from build123d import *

# Parameters (mm, degrees)
F1_DEPTH = 6.35


with BuildPart() as f1:
    # F0 (on Front) → F1 (new body)
    with BuildSketch(Plane.XZ):
        with BuildLine():
            Line((254, 6.35), (0, 6.35))
            Line((0, 6.35), (0, 0))
            ThreePointArc((0, 0), (2.54, -2.54), (5.08, 0))
            Line((5.08, 0), (5.6896, 0))
            ThreePointArc((5.6896, 0), (8.2296, -2.54), (10.7696, 0))
            Line((10.7696, 0), (11.3792, 0))
            ThreePointArc((11.3792, 0), (13.9192, -2.54), (16.4592, 0))
            Line((16.4592, 0), (17.0688, 0))
            ThreePointArc((17.0688, 0), (19.6088, -2.54), (22.1488, 0))
            Line((22.1488, 0), (22.7584, 0))
            ThreePointArc((22.7584, 0), (25.2984, -2.54), (27.8384, 0))
            Line((27.8384, 0), (28.448, 0))
            ThreePointArc((28.448, 0), (30.988, -2.54), (33.528, 0))
            Line((33.528, 0), (34.1376, 0))
            ThreePointArc((34.1376, 0), (36.6776, -2.54), (39.2176, 0))
            Line((39.2176, 0), (39.8272, 0))
            ThreePointArc((39.8272, 0), (42.3672, -2.54), (44.9072, 0))
            Line((44.9072, 0), (45.5168, 0))
            ThreePointArc((45.5168, 0), (48.0568, -2.54), (50.5968, 0))
            Line((50.5968, 0), (51.2064, 0))
            ThreePointArc((51.2064, 0), (53.7464, -2.54), (56.2864, 0))
            Line((56.2864, 0), (56.896, 0))
            ThreePointArc((56.896, 0), (59.436, -2.54), (61.976, 0))
            Line((61.976, 0), (62.5856, 0))
            ThreePointArc((62.5856, 0), (65.1256, -2.54), (67.6656, 0))
            Line((67.6656, 0), (68.2752, 0))
            ThreePointArc((68.2752, 0), (70.8152, -2.54), (73.3552, 0))
            Line((73.3552, 0), (73.9648, 0))
            ThreePointArc((73.9648, 0), (76.5048, -2.54), (79.0448, 0))
            Line((79.0448, 0), (79.6544, 0))
            ThreePointArc((79.6544, 0), (82.1944, -2.54), (84.7344, 0))
            Line((84.7344, 0), (85.344, 0))
            ThreePointArc((85.344, 0), (87.884, -2.54), (90.424, 0))
            Line((90.424, 0), (91.0336, 0))
            ThreePointArc((91.0336, 0), (93.5736, -2.54), (96.1136, 0))
            Line((96.1136, 0), (96.7232, 0))
            ThreePointArc((96.7232, 0), (99.2632, -2.54), (101.8032, 0))
            Line((101.8032, 0), (102.4128, 0))
            ThreePointArc((102.4128, 0), (104.9528, -2.54), (107.4928, 0))
            Line((107.4928, 0), (108.1024, 0))
            ThreePointArc((108.1024, 0), (110.6424, -2.54), (113.1824, 0))
            Line((113.1824, 0), (113.792, 0))
            ThreePointArc((113.792, 0), (116.332, -2.54), (118.872, 0))
            Line((118.872, 0), (119.4816, 0))
            ThreePointArc((119.4816, 0), (122.0216, -2.54), (124.5616, 0))
            Line((124.5616, 0), (125.1712, 0))
            ThreePointArc((125.1712, 0), (127.7112, -2.54), (130.2512, 0))
            Line((130.2512, 0), (130.8608, 0))
            ThreePointArc((130.8608, 0), (133.4008, -2.54), (135.9408, 0))
            Line((135.9408, 0), (136.5504, 0))
            ThreePointArc((136.5504, 0), (139.0904, -2.54), (141.6304, 0))
            Line((141.6304, 0), (142.24, 0))
            ThreePointArc((142.24, 0), (144.78, -2.54), (147.32, 0))
            Line((147.32, 0), (147.9296, 0))
            ThreePointArc((147.9296, 0), (150.4696, -2.54), (153.0096, 0))
            Line((153.0096, 0), (153.6192, 0))
            ThreePointArc((153.6192, 0), (156.1592, -2.54), (158.6992, 0))
            Line((158.6992, 0), (159.3088, 0))
            ThreePointArc((159.3088, 0), (161.8488, -2.54), (164.3888, 0))
            Line((164.3888, 0), (164.9984, 0))
            ThreePointArc((164.9984, 0), (167.5384, -2.54), (170.0784, 0))
            Line((170.0784, 0), (170.688, 0))
            ThreePointArc((170.688, 0), (173.228, -2.54), (175.768, 0))
            Line((175.768, 0), (176.3776, 0))
            ThreePointArc((176.3776, 0), (178.9176, -2.54), (181.4576, 0))
            Line((181.4576, 0), (182.0672, 0))
            ThreePointArc((182.0672, 0), (184.6072, -2.54), (187.1472, 0))
            Line((187.1472, 0), (187.7568, 0))
            ThreePointArc((187.7568, 0), (190.2968, -2.54), (192.8368, 0))
            Line((192.8368, 0), (193.4464, 0))
            ThreePointArc((193.4464, 0), (195.9864, -2.54), (198.5264, 0))
            Line((198.5264, 0), (199.136, 0))
            ThreePointArc((199.136, 0), (201.676, -2.54), (204.216, 0))
            Line((204.216, 0), (204.8256, 0))
            ThreePointArc((204.8256, 0), (207.3656, -2.54), (209.9056, 0))
            Line((209.9056, 0), (210.5152, 0))
            ThreePointArc((210.5152, 0), (213.0552, -2.54), (215.5952, 0))
            Line((215.5952, 0), (216.2048, 0))
            ThreePointArc((216.2048, 0), (218.7448, -2.54), (221.2848, 0))
            Line((221.2848, 0), (221.8944, 0))
            ThreePointArc((221.8944, 0), (224.4344, -2.54), (226.9744, 0))
            Line((226.9744, 0), (227.584, 0))
            ThreePointArc((227.584, 0), (230.124, -2.54), (232.664, 0))
            Line((232.664, 0), (233.2736, 0))
            ThreePointArc((233.2736, 0), (235.8136, -2.54), (238.3536, 0))
            Line((238.3536, 0), (238.9632, 0))
            ThreePointArc((238.9632, 0), (241.5032, -2.54), (244.0432, 0))
            Line((244.0432, 0), (244.6528, 0))
            ThreePointArc((244.6528, 0), (247.1928, -2.54), (249.7328, 0))
            Line((249.7328, 0), (254, 0))
            Line((254, 0), (254, 6.35))
        make_face()
    extrude(amount=F1_DEPTH)


solid = f1.part
Work out the finished part from the listing and answer in its coordinate system (mm). Round coordinates to 2 decimals unless told otherwise and drop trailing zeros. Answer as CSV lines item,"result". Start each with the question number.
(1) Find the intervals of material crossed by probe 1 along Z at (x, y) = (99, -2); probe 2 along Z at (x, y) = (45, -0.5), in increasing order.
(2) Each of these flat-tipped pins is pushed along its axis until it touches: pin 1 (0.7 mm diameter, centred on x = 153, y = -3, fed in from -Z); pin 2 (0.7 mm diameter, centred on x = 227.5, y = -3.5, fed in from -Z); pin 3 (4 mm diameter, centred on x = 182.5, z = 1.5, fed in from +Y). Where does it stop, or does it pass through?
(3) The mould has two halves that part along X. Classify faces 1 (the cylindrical face through (224.38, -3.13, -2.54)), 2 (the cylindrical face through (235.76, -3.13, -2.54)): +X half, -X half, draft (parallel to the pull), parting line (faces both ways), or undercut.
Output values:
1,probe 1,"z = -2.53 to 6.35"
1,probe 2,"z = 0 to 6.35"
2,pin 1,"stops at z = -1.3"
2,pin 2,"stops at z = -1.13"
2,pin 3,"stops at y = 0"
3,face 1,"undercut"
3,face 2,"undercut"
